Check sheet for the modelled part. Datum: model origin and axes. Units: mm. Face numbers are marked on the shaded views. A direction names the side the tool comes from. Give positions to 0.01 mm unless a question says otherwise; leave off trailing zeros. Order: outer loops, then holes, each group sorted by start corner. A loop starts at its lowest first (then second) coordinate and runs counter-clockwise, first axis right, second up.
Item 1: Sectioned sample at D-D on x = 62.5. Record the boundary of the cut face in (y, z), and give its area (3 significant figures).
Item 2: Sectioned sample at C-C on z = -101.5. Record the boundary of the cut face in (x, y).
Item 3: Release check for a two-part mould opening along Z. For the marked faces 1, 2 and 3 record: released by +Z, released by -Z, zero draft, split by the parting line, or undercut.
Item 4: Material ranges on line 1 along X through (y, z) = (44, -165); line 2 along Y through (x, z) = (-47.5, -139); line 3 along Z through (x, y) = (58, 64.5), recorded low to high.
Item 5: Gauge pin test, flat ends, axial feed: P1, Ø12, axis at x = -6, z = -139.5, coming from the -Y side; P2, Ø12, axis at y = 68, z = -133, coming from the +X side. Record the tip position at first contact, or that the pin passes through.
Item 6: Sectioned sample at B-B on x = 41. Record the boundary of the cut face in (y, z), and give its area (3 significant figures).
Item 7: Sectioned sample at A-A on y = 93. Record the boundary of the cut face in (x, z).
Item 8: Access from +Z, -Z, +X, -X, +Y, -Y to the whole of each face (thin tool, end or side, straight path). Record for the marked faces 4, 5, 6, 7 and 8.
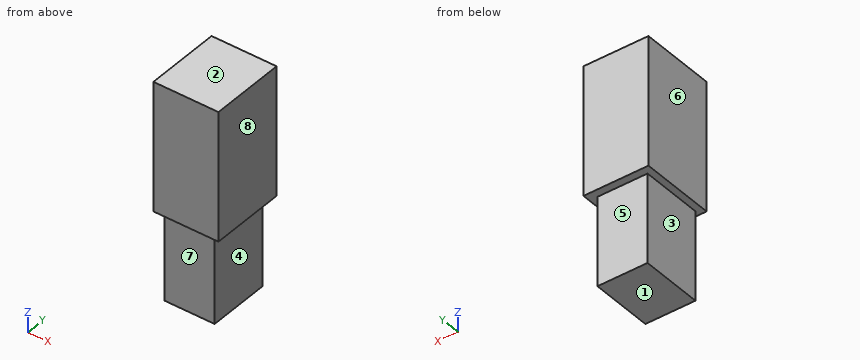
from build123d import *

# Parameters (mm, degrees)
F0_W     = 145.7732766867
F0_H     = 72.8164315224
F1_DEPTH = 169.5371419191
F2_DEPTH = 25.4
F3_DEPTH = 191.2825796753
F4_W     = 112.2992113233
F4_H     = 139.7446542978
F5_DEPTH = 489.1429543495


with BuildPart() as f1:
    # F0 (on Front) → F1 (new body)
    with BuildSketch(Plane.XZ):
        with Locations((0.2535507083, -36.4082157612)):
            Rectangle(F0_W, F0_H)
    extrude(amount=-F1_DEPTH)

    # F2 (add): a face of the model
    f2_faces = [f1.faces().sort_by_distance(p)[0] for p in [
        (0.2535507083, 84.7685709596, 0),
    ]]
    extrude(f2_faces, amount=F2_DEPTH)

    # F3 (add): a face of the model
    f3_faces = [f1.faces().sort_by_distance(p)[0] for p in [
        (0.2535507083, 84.7685709596, 25.4),
    ]]
    extrude(f3_faces, amount=F3_DEPTH)

    # F4 (on face) → F5 (join)
    with BuildSketch(Plane.XY.offset(216.6825796753)):
        with Locations((-1.0879933834, 82.2958871722)):
            Rectangle(F4_W, F4_H)
    extrude(amount=-F5_DEPTH)


solid = f1.part
Report:
1. outline: (0, -72.82) - (169.54, -72.82) - (169.54, 216.68) - (0, 216.68) - close
1. area: 49,100 mm2
2. outline: (-57.24, 12.42) - (55.06, 12.42) - (55.06, 152.17) - (-57.24, 152.17) - close
3. face 1: released by -Z
3. face 2: released by +Z
3. face 3: zero draft
4. line 1: x = -57.24 to 55.06
4. line 2: y = 12.42 to 152.17
4. line 3: z = -72.82 to 216.68
5. P1: stops at y = 12.42
5. P2: stops at x = 55.06
6. outline: (0, -72.82) - (12.42, -72.82) - (12.42, -272.46) - (152.17, -272.46) - (152.17, -72.82) - (169.54, -72.82) - (169.54, 216.68) - (0, 216.68) - close
6. area: 77,000 mm2
7. outline: (-72.63, -72.82) - (-57.24, -72.82) - (-57.24, -272.46) - (55.06, -272.46) - (55.06, -72.82) - (73.14, -72.82) - (73.14, 216.68) - (-72.63, 216.68) - close
8. face 4: -Z, +X, +Y, -Y
8. face 5: -Z, +X, -X, +Y
8. face 6: +Z, -Z, -X, +Y, -Y
8. face 7: -Z, +X, -X, -Y
8. face 8: +Z, -Z, +X, +Y, -Y
